Here's how the part is built. I have some questions about the finished solid (model axes, mm). A direction names the side the tool comes from. Coordinates: 2 decimals unless noted, no trailing zeros. Loops run counter-clockwise (first coordinate to the right, second up) from the corner with the lowest first, then second, coordinate; pieces in that order, holes last.
Autodesk Inventor part; units mm, degrees
ref_plane "YZ Plane" through (0, 0, 0) normal (1, 0, 0) x (0, 1, 0)
ref_plane "XZ Plane" through (0, 0, 0) normal (0, 1, 0) x (-1, 0, 0)
ref_plane "XY Plane" through (0, 0, 0) normal (0, 0, 1) x (1, 0, 0)
sketch "Эскиз1" plane through (0, 0, 0) normal (0, 1, 0) x (-1, 0, 0)
  line L0 (0, 0) -> (9.1667, 0)
  line L1 (0, 0) -> (0, -12.5)
  line L2 (-11.2667, 28.6) -> (11.2667, 28.6)
  line L3 (18.2667, 21.6) -> (18.2667, -21.6)
  line L4 (-18.2667, -21.6) -> (-18.2667, 21.6)
  line L5 (13.1667, -2.1) -> (16.2667, -2.1)
  line L6 (16.2667, -2.1) -> (16.2667, -20.7)
  line L7 (16.2667, -20.7) -> (13.1667, -20.7)
  line L8 (13.1667, 2.1) -> (16.2667, 2.1)
  line L9 (16.2667, 2.1) -> (16.2667, 20.7)
  line L10 (16.2667, 20.7) -> (13.1667, 20.7)
  line L11 (-16.2667, 2.1) -> (-16.2667, 20.7)
  line L12 (-16.2667, 20.7) -> (-13.1667, 20.7)
  line L13 (-13.1667, 2.1) -> (-16.2667, 2.1)
  line L14 (-13.1667, -2.1) -> (-16.2667, -2.1)
  line L15 (-16.2667, -2.1) -> (-16.2667, -20.7)
  line L16 (-16.2667, -20.7) -> (-13.1667, -20.7)
  line L17 (10.1667, -23.5) -> (10.1667, -26.6)
  line L18 (-10.1667, -26.6) -> (-10.1667, -23.5)
  line L19 (10.1667, 23.5) -> (10.1667, 26.6)
  line L20 (10.1667, 26.6) -> (-10.1667, 26.6)
  line L21 (-10.1667, 26.6) -> (-10.1667, 23.5)
  arc A0 (18.2667, 21.6) -> (11.2667, 28.6) centre (11.2667, 21.6) ccw
  arc A1 (-11.2667, 28.6) -> (-18.2667, 21.6) centre (-11.2667, 21.6) ccw
  arc A2 (-18.2667, -21.6) -> (-11.2667, -28.6) centre (-11.2667, -21.6) ccw
  arc A3 (11.2667, -28.6) -> (18.2667, -21.6) centre (11.2667, -21.6) ccw
  line L22 (-10.1667, -26.6) -> (-10.1667, -28.6)
  line L23 (-10.1667, -28.6) -> (-11.2667, -28.6)
  line L24 (10.1667, -26.6) -> (10.1667, -28.6)
  line L25 (10.1667, -28.6) -> (11.2667, -28.6)
  line L26 (-10.1667, 23.5) -> (-13.1667, 23.5)
  line L27 (-13.1667, 23.5) -> (-13.1667, 20.7)
  line L28 (10.1667, 23.5) -> (13.1667, 23.5)
  line L29 (13.1667, 23.5) -> (13.1667, 20.7)
  line L30 (-10.1667, -23.5) -> (-13.1667, -23.5)
  line L31 (-13.1667, -23.5) -> (-13.1667, -20.7)
  line L32 (10.1667, -23.5) -> (13.1667, -23.5)
  line L33 (13.1667, -23.5) -> (13.1667, -20.7)
  line L34 (13.1667, 2.1) -> (13.1667, -2.1)
  line L35 (-13.1667, 2.1) -> (-13.1667, -2.1)
extrude "Выдавливание1" add sketch "Эскиз1" along normal blind 4.5
sketch "Эскиз2" plane through (-13.1667, 0, 2.1) normal (1, 0, 0) x (0, 0, -1)
  line L0 (-18.6, 0) -> (0, 0)
  line L1 (4.2, 0) -> (4.2, 4.5)
  line L2 (0, 0) -> (4.2, 0)
  line L3 (4.2, 0) -> (4.2, 2)
  line L4 (4.2, 2) -> (0, 2)
  line L5 (0, 2) -> (0, 0)
  point P0 (2.1, 0)
  dimension "d19" = 2
extrude "Выдавливание2" add sketch "Эскиз2" along normal blind 1
chamfer "Фаска1" distance 1.8 angle 45 1 edges at (-12.1667, 0, 0)
mirror "Зеркальное отражение1" about plane through (0, 0, 0) normal (1, 0, 0) of "Выдавливание2", "Фаска1"
sketch "Эскиз3" plane through (-11.2667, 0, 28.6) normal (0, 0, 1) x (1, 0, 0)
  line L0 (1.1, 4.5) -> (-1.9, 4.5)
  line L1 (21.4333, 0) -> (24.4333, 0)
  line L2 (-0.4, 4.5) -> (22.9333, 4.5)
  line L3 (22.9333, 4.5) -> (22.9333, 0)
  line L4 (22.9333, 0) -> (-0.4, 0)
  line L5 (-0.4, 0) -> (-0.4, 4.5)
  point P0 (11.2667, 0)
extrude "Выдавливание3" add sketch "Эскиз3" along normal blind 7.9
sketch "Эскиз4" plane through (0, 4.5, 0) normal (0, 1, 0) x (1, 0, 0)
  line L0 (-11.2667, -28.6) -> (-11.6667, -28.6)
  line L1 (11.6667, -36.5) -> (-11.6667, -36.5)
  line L2 (-11.6667, -28.6) -> (11.6667, -28.6)
  line L3 (11.6667, -28.6) -> (11.6667, -36.5)
  line L4 (11.6667, -36.5) -> (-11.6667, -36.5)
  line L5 (-11.6667, -36.5) -> (-11.6667, -28.6)
  point P0 (0, 0)
extrude "Выдавливание4" add sketch "Эскиз4" against normal blind 21
sketch "Эскиз5" plane through (0, 4.5, 0) normal (0, 1, 0) x (1, 0, 0)
  line L0 (-10.6667, -35.5) -> (10.6667, -35.5)
  line L1 (10.6667, -35.5) -> (10.6667, -29.6)
  line L2 (10.6667, -29.6) -> (-10.6667, -29.6)
  line L3 (-10.6667, -29.6) -> (-10.6667, -35.5)
  line L4 (-11.6667, -28.6) -> (-11.6667, -36.5)
  line L5 (11.6667, -28.6) -> (11.6667, -36.5)
  line L6 (11.6667, -36.5) -> (-11.6667, -36.5)
  line L7 (11.2667, -28.6) -> (-11.2667, -28.6)
  point P0 (0, 0)
  dimension "d29" = 1
  dimension "d30" = 1
  dimension "d31" = 1
  dimension "d32" = 1
extrude "Выдавливание5" cut sketch "Эскиз5" against normal blind 20
sketch "Эскиз6" plane through (0, 4.5, 0) normal (0, 1, 0) x (1, 0, 0)
  line L0 (-11.6667, -28.6) -> (-11.6667, -36.5)
  line L1 (11.6667, -28.6) -> (11.2667, -28.6)
  line L2 (-11.6667, -28.6) -> (11.6667, -28.6)
  line L3 (-11.6667, -28.6) -> (-11.6667, -36.5)
  line L4 (11.6667, -36.5) -> (-11.6667, -36.5)
  line L5 (11.6667, -28.6) -> (11.6667, -36.5)
  line L6 (11.6667, -36.5) -> (11.6667, -28.6)
  line L7 (11.6667, -36.5) -> (-11.6667, -36.5)
  line L8 (-10.6667, -29.6) -> (10.6667, -29.6)
  line L9 (10.6667, -29.6) -> (10.6667, -35.5)
  line L10 (-10.6667, -29.6) -> (10.6667, -29.6)
  line L11 (10.6667, -29.6) -> (10.6667, -35.5)
  line L12 (10.6667, -35.5) -> (-10.6667, -35.5)
  line L13 (-10.6667, -35.5) -> (-10.6667, -29.6)
  point P0 (0, 0)
extrude "Выдавливание6" add sketch "Эскиз6" along normal blind 8
sketch "Эскиз7" plane through (0, 12.5, 0) normal (0, 1, 0) x (1, 0, 0)
  line L0 (-11.6667, -36.5) -> (-11.6667, -28.6)
  line L1 (11.6667, -36.5) -> (-11.6667, -36.5)
  line L2 (-11.6667, -28.6) -> (11.6667, -28.6)
  line L3 (11.6667, -28.6) -> (11.6667, -36.5)
  line L4 (11.6667, -36.5) -> (-11.6667, -36.5)
  line L5 (-11.6667, -36.5) -> (-11.6667, -28.6)
  line L6 (10.6667, -29.6) -> (10.6667, -35.5)
  line L7 (-10.6667, -35.5) -> (-10.6667, -29.6)
  line L8 (11.2667, -28.6) -> (-11.2667, -28.6)
  line L9 (-1.6667, -28.6) -> (1.6667, -28.6)
  line L10 (-10.6667, -29.6) -> (-11.6667, -29.6)
  line L11 (-10.6667, -35.5) -> (-11.6667, -35.5)
  line L12 (10.6667, -35.5) -> (11.6667, -35.5)
  line L13 (10.6667, -29.6) -> (11.6667, -29.6)
  line L14 (1.6667, -36.5) -> (-1.6667, -36.5)
  line L15 (-10.6667, -35.5) -> (-10.6667, -29.6)
  line L16 (-10.6667, -29.6) -> (-10.6667, -29.4)
  line L17 (-10.6667, -29.4) -> (10.6667, -29.4)
  line L18 (10.6667, -29.4) -> (10.6667, -29.6)
  line L19 (-10.6667, -35.5) -> (-10.6667, -35.7)
  line L20 (-10.6667, -35.7) -> (10.6667, -35.7)
  line L21 (10.6667, -35.7) -> (10.6667, -35.5)
  line L22 (-1.6667, -28.6) -> (1.6667, -28.6)
  line L23 (1.6667, -28.6) -> (1.6667, -29.4)
  line L24 (1.6667, -29.4) -> (-1.6667, -29.4)
  line L25 (-1.6667, -29.4) -> (-1.6667, -28.6)
  line L26 (-1.6667, -35.7) -> (1.6667, -35.7)
  line L27 (1.6667, -35.7) -> (1.6667, -36.5)
  line L28 (1.6667, -36.5) -> (-1.6667, -36.5)
  line L29 (-1.6667, -36.5) -> (-1.6667, -35.7)
  point P0 (0, 0)
  dimension "d42" = 0.8
  dimension "d43" = 0.8
  dimension "d44" = 10
  dimension "d45" = 10
  dimension "d46" = 10
  dimension "d47" = 10
extrude "Выдавливание7" add sketch "Эскиз7" along normal blind 4 contours L0 L11 L19 L20 L29 L1 | L0 L2 L25 L17 L16 L10 | L27 L20 L21 L12 L3 L1 | L13 L18 L17 L23 L2 L3
sketch "Эскиз8" plane through (0, 16.5, 0) normal (0, 1, 0) x (1, 0, 0)
  line L0 (-11.6667, -28.6) -> (-11.6667, -29.6)
  line L1 (11.6667, -36.5) -> (-11.6667, -36.5)
  line L2 (-11.6667, -28.6) -> (11.6667, -28.6)
  line L3 (11.6667, -28.6) -> (11.6667, -36.5)
  line L4 (11.6667, -36.5) -> (-11.6667, -36.5)
  line L5 (-11.6667, -36.5) -> (-11.6667, -28.6)
  line L6 (-10.6667, -29.4) -> (-1.6667, -29.4)
  line L7 (10.6667, -35.7) -> (1.6667, -35.7)
  line L8 (-10.6667, -29.4) -> (10.6667, -29.4)
  line L9 (10.6667, -29.4) -> (10.6667, -35.7)
  line L10 (10.6667, -35.7) -> (-10.6667, -35.7)
  line L11 (-10.6667, -35.7) -> (-10.6667, -29.4)
  point P0 (0, 0)
extrude "Выдавливание8" add sketch "Эскиз8" against normal blind 1.8
properties part number "Extension"
1. For pin 1 (2 mm diameter, centred on x = -13, z = 2, fed in from +Y); pin 2 (12 mm diameter, centred on x = -1, y = -8, fed in from -Z); pin 3 (0.9 mm diameter, centred on x = 14.5, y = 3, fed in from +Z), each with a flat end and sliding along its axis, tell me the tip position at first contact or that it passes through.
2. I want a section at D-D (x = -8). Please give me the cut outline in (y, z), then the cut area to 3 significant figures.
3. On a 3-axis mill with a long thin cutter (end or side, diameter ignored), from which of +Z, -Z, +X, -X, +Y, -Y can I reach the whole of each face in a straight line? I mean faces 1 (the flat face through (15, 2, -20.7)), 2 (the flat face through (-15, 0, 0)), 3 (the flat face through (13.167, 3, 0)). Say none if no direction works.
4. We'd pull the mould along X, two halves only. Please class faces 4 (the cylindrical face through (16.162, 2.218, -26.604)), 5 (the flat face through (0, -2, 35.5)), 6 (the cylindrical face through (-16.271, 2.218, -26.495)): +X half, -X half, draft (parallel to the pull), parting line (faces both ways), or undercut.
5. I want a section at A-A (x = 0.5). Please give me the cut outline in (y, z), then the cut area to 3 significant figures.
6. I want a section at B-B (y = 10.5). Please give me the cut outline in (x, z).
7. I want a section at C-C (z = -19). Please give me the cut outline in (x, y), then the cut area to 3 significant figures.
8. I need wall thicknesses on line 1 along Z through (x, y) = (-2.5, -13); line 2 along X through (y, z) = (3, -1.5); line 3 along X through (y, z) = (-8.5, 32.5). Which ranges of each line are inside material? Lowest first, please.
Response values:
1. pin 1: stops at y = 4.5
1. pin 2: stops at z = 28.6
1. pin 3: stops at z = 28.02
2. outline: (-16.5, 28.6) - (0, 28.6) - (0, 26.6) - (4.5, 26.6) - (4.5, 28.6) - (16.5, 28.6) - (16.5, 29.4) - (12.5, 29.4) - (12.5, 29.6) - (-15.5, 29.6) - (-15.5, 35.5) - (12.5, 35.5) - (12.5, 35.7) - (16.5, 35.7) - (16.5, 36.5) - (-16.5, 36.5) - close
2. area: 79.3 mm2
3. face 1: +Y, -Y
3. face 2: -Z, +X, -X, -Y
3. face 3: +Y
4. face 4: +X half
4. face 5: undercut
4. face 6: -X half
5. outline: (-16.5, 28.6) - (0, 28.6) - (0, 26.6) - (4.5, 26.6) - (4.5, 28.6) - (12.5, 28.6) - (12.5, 29.6) - (-15.5, 29.6) - (-15.5, 35.5) - (12.5, 35.5) - (12.5, 36.5) - (-16.5, 36.5) - close; (14.7, 28.6) - (16.5, 28.6) - (16.5, 29.4) - (14.7, 29.4) - close; (14.7, 35.7) - (16.5, 35.7) - (16.5, 36.5) - (14.7, 36.5) - close
5. area: 75.8 mm2
6. outline: (-11.67, 28.6) - (11.67, 28.6) - (11.67, 36.5) - (-11.67, 36.5) - close; hole (-10.67, 29.6) - (10.67, 29.6) - (10.67, 35.5) - (-10.67, 35.5) - close
7. outline: (-18.27, 0) - (-16.27, 0) - (-16.27, 4.5) - (-18.27, 4.5) - close; (16.27, 0) - (18.27, 0) - (18.27, 4.5) - (16.27, 4.5) - close
7. area: 18.0 mm2
8. line 1: z = 28.6 to 29.6, 35.5 to 36.5
8. line 2: x = -18.27 to -13.17, 13.17 to 18.27
8. line 3: x = -11.67 to -10.67, 10.67 to 11.67
